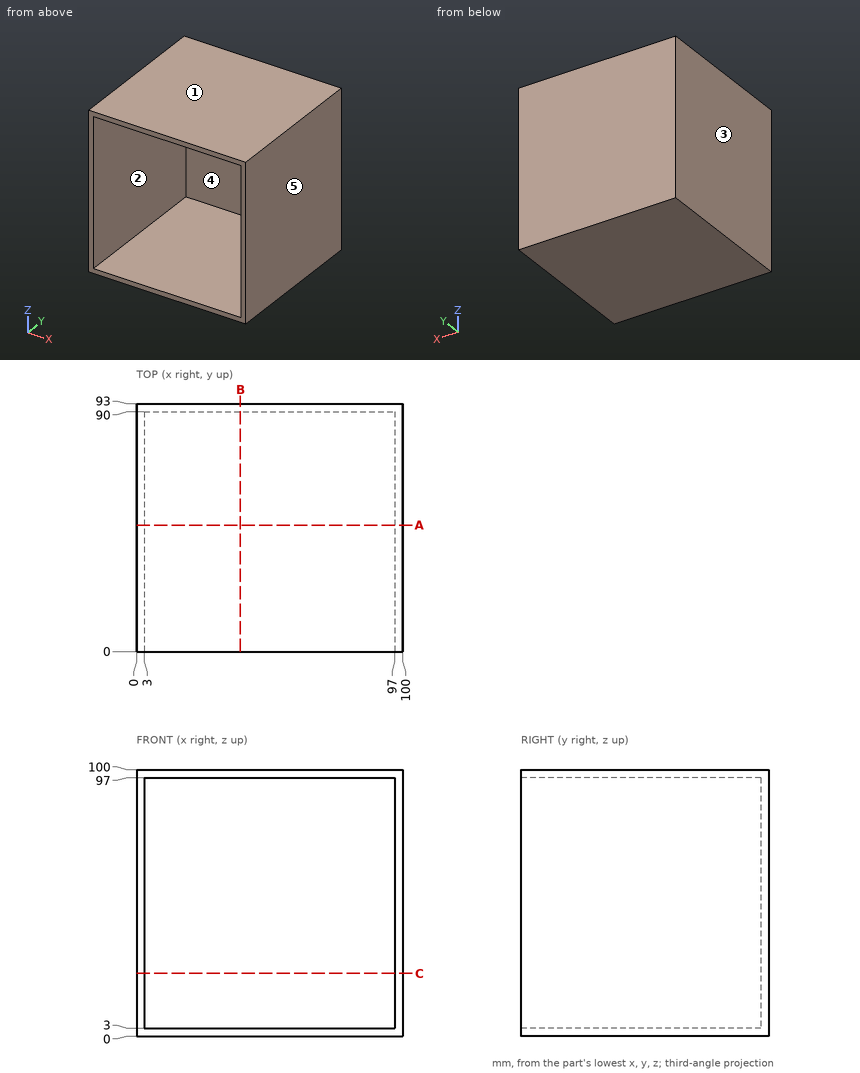
Input: dimensioned drawing with shaded views. Units: mm. Origin: part minimum x, y, z. A direction names the side the tool comes from. Round coordinates to 2 decimals unless told otherwise and drop trailing zeros. Order: outer loops, then holes, each group sorted by start corner. A loop starts at its lowest first (then second) coordinate and runs counter-clockwise, first axis right, second up. Notation, with made-up numbers: (36, 68) -> (73, 68) arc R30 cw to (73, 102) -> close; hole circle Ø2 at (17, -9). An arc over 180 degrees is marked (long way). Put each result on its own line as item: value. Start each with the question number.
Q1. Section A-A on y = 47.5. Return the cut outline in (x, z).
Q2. Pull-direction query (X, two-part tool) for the marked faces 3, 4 and 5; classes: +X half, -X half, draft (parallel to the pull), parting line (faces both ways), or undercut.
Q3. Section C-C on z = 23.5. Return the cut outline in (x, y), and give its area (3 significant figures).
Q4. Line query: probe 1 along X at (y, z) = (86, 23); probe 2 along Y at (x, z) = (60, 70). Output: solid intervals per line, ascending.
Q5. Reachability of the marked faces 1 and 2 from +Z, -Z, +X, -X, +Y, -Y: full face, straight path, thin tool, end or side. Return the list, or none.
Q6. Section B-B on x = 39. Return the cut outline in (y, z), and give its area (3 significant figures).
Q7. First-contact query: pin 1 (8 mm diameter, centred on x = 29, z = 74.5, fed in from -Y). Flat tip, straight axial feed; report the tip coordinate or a pass-through.
Ans:
1. outline: (0, 0) -> (100, 0) -> (100, 100) -> (0, 100) -> close; hole (3, 3) -> (97, 3) -> (97, 97) -> (3, 97) -> close
2. face 3: -X half
2. face 4: undercut
2. face 5: +X half
3. outline: (0, 0) -> (3, 0) -> (3, 90) -> (97, 90) -> (97, 0) -> (100, 0) -> (100, 93) -> (0, 93) -> close
3. area: 840 mm2
4. probe 1: x = 0 to 3, 97 to 100
4. probe 2: y = 90 to 93
5. face 1: +Z, +X, -X, +Y, -Y
5. face 2: -Y
6. outline: (0, 0) -> (93, 0) -> (93, 100) -> (0, 100) -> (0, 97) -> (90, 97) -> (90, 3) -> (0, 3) -> close
6. area: 840 mm2
7. pin 1: stops at y = 90
